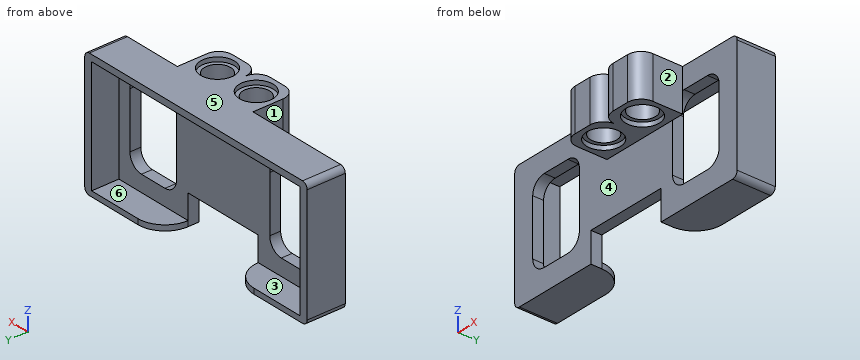
from build123d import *

# Parameters (mm, degrees)
SKETCH1_W           = 48.2
SKETCH1_H           = 23.2
BOSS_EXTRUDE1_DEPTH = 10
SKETCH2_W           = 46.2
SKETCH2_H           = 21.2
CUT_EXTRUDE1_DEPTH  = 8
SKETCH3_W           = 11.2
SKETCH3_H           = 5
CUT_EXTRUDE2_DEPTH  = 10
SKETCH4_W           = 48.2
SKETCH4_H           = 23.2
CUT_EXTRUDE3_DEPTH  = 3
SKETCH5_W           = 8.2
SKETCH5_H           = 7.76
BOSS_EXTRUDE2_DEPTH = 8
SKETCH6_R           = 3.1
CUT_EXTRUDE4_DEPTH  = 0.8
SKETCH7_R           = 2.4
CUT_EXTRUDE5_DEPTH  = 10
SKETCH8_W           = 46.2
SKETCH8_H           = 20.3
CUT_EXTRUDE6_DEPTH  = 5
SKETCH9_W           = 45.4
SKETCH9_H           = 20.3
CUT_EXTRUDE8_DEPTH  = 5
CUT_EXTRUDE9_START  = -0.8
SKETCH10_R          = 3.1
CUT_EXTRUDE9_DEPTH  = 0.8
SKETCH11_W          = 15.2
SKETCH11_H          = 5.5
CUT_EXTRUDE10_DEPTH = 10
CUT_EXTRUDE11_DEPTH = 10
FILLET1_R           = 1
FILLET2_R           = 1
FILLET3_R           = 1
FILLET4_R           = 1
FILLET5_R           = 2.5
FILLET6_R           = 2.5
FILLET7_R           = 5
FILLET8_R           = 5
SKETCH13_W          = 21.2
SKETCH13_H          = 5
BOSS_EXTRUDE3_DEPTH = 0.5
SKETCH14_W          = 21.2
SKETCH14_H          = 5
BOSS_EXTRUDE4_DEPTH = 0.5
SKETCH16_W          = 45.2
SKETCH16_H          = 5
BOSS_EXTRUDE5_DEPTH = 0.2
MIRROR4_START       = 13.310407833
MIRROR4_OUTLINE_R   = 2.4
MIRROR4_DEPTH       = 6.16
MIRROR4_START_2     = 12.510407833
MIRROR4_2_OUTLINE_R = 3.1
MIRROR4_2_DEPTH     = 7.76


# Read off the part's stored shape, not the designer's step: Mirror4
with BuildPart() as part:
    # Sketch1 → Boss-Extrude1 (new body)
    with BuildSketch(Plane(origin=(0, 0, 0), x_dir=(1, 0, 0), z_dir=(0, 1, 0))):
        with Locations((-8.956036835, -8.670407833)):
            Rectangle(SKETCH1_W, SKETCH1_H)
    extrude(amount=BOSS_EXTRUDE1_DEPTH)

    # Sketch2 → Cut-Extrude1 (cut)
    with BuildSketch(Plane(origin=(0, 10, 0), x_dir=(1, 0, 0), z_dir=(0, 1, 0))):
        with Locations((-8.956036835, -8.670407833)):
            Rectangle(SKETCH2_W, SKETCH2_H)
    extrude(amount=-CUT_EXTRUDE1_DEPTH, mode=Mode.SUBTRACT)

    # Sketch3 → Cut-Extrude2 (cut)
    with BuildSketch(Plane(origin=(0, 10, 0), x_dir=(1, 0, 0), z_dir=(0, 1, 0))):
        with Locations((-8.956036835, 0.429592167)):
            Rectangle(SKETCH3_W, SKETCH3_H)
    extrude(amount=-CUT_EXTRUDE2_DEPTH, mode=Mode.SUBTRACT)

    # Sketch4 → Cut-Extrude3 (cut)
    with BuildSketch(Plane(origin=(0, 10, 0), x_dir=(1, 0, 0), z_dir=(0, 1, 0))):
        with Locations((-8.956036835, -8.670407833)):
            Rectangle(SKETCH4_W, SKETCH4_H)
    extrude(amount=-CUT_EXTRUDE3_DEPTH, mode=Mode.SUBTRACT)

    # Sketch5 → Boss-Extrude2 (add)
    with BuildSketch(Plane(origin=(0, 0, 0), x_dir=(-1, 0, 0), z_dir=(0, -1, 0))):
        with Locations((8.956036835, -16.390407833)):
            Rectangle(SKETCH5_W, SKETCH5_H)
    extrude(amount=BOSS_EXTRUDE2_DEPTH)

    # Sketch6 → Cut-Extrude4 (cut)
    with BuildSketch(Plane.XY.offset(20.270407833)):
        with Locations((-9.056036835, -4)):
            Circle(SKETCH6_R)
    extrude(amount=-CUT_EXTRUDE4_DEPTH, mode=Mode.SUBTRACT)

    # Sketch7 → Cut-Extrude5 (cut)
    with BuildSketch(Plane.XY.offset(19.470407833)):
        with Locations((-9.056036835, -4)):
            Circle(SKETCH7_R)
    extrude(amount=-CUT_EXTRUDE5_DEPTH, mode=Mode.SUBTRACT)

    # Sketch8 → Cut-Extrude6 (cut)
    with BuildSketch(Plane(origin=(0, 7, 0), x_dir=(1, 0, 0), z_dir=(0, 1, 0))):
        with Locations((-8.956036835, -8.720407833)):
            Rectangle(SKETCH8_W, SKETCH8_H)
    extrude(amount=-CUT_EXTRUDE6_DEPTH, mode=Mode.SUBTRACT)

    # Sketch9 → Cut-Extrude8 (cut)
    with BuildSketch(Plane(origin=(0, 7, 0), x_dir=(1, 0, 0), z_dir=(0, 1, 0))):
        with Locations((-8.956036835, -8.720407833)):
            Rectangle(SKETCH9_W, SKETCH9_H)
    extrude(amount=-CUT_EXTRUDE8_DEPTH, mode=Mode.SUBTRACT)

    # Sketch10 → Cut-Extrude9 (cut)
    with BuildSketch(Plane(origin=(0, 0, 12.510407833), x_dir=(-1, 0, 0), z_dir=(0, 0, -1)).offset(CUT_EXTRUDE9_START)):
        with Locations(Location((9.056036835, -4, 0), (0, 0, 180))):
            Circle(SKETCH10_R)
    extrude(amount=CUT_EXTRUDE9_DEPTH, mode=Mode.SUBTRACT)

    # Sketch11 → Cut-Extrude10 (cut)
    with BuildSketch(Plane(origin=(0, 7, 0), x_dir=(1, 0, 0), z_dir=(0, 1, 0))):
        with Locations((-8.956036835, 0.179592167)):
            Rectangle(SKETCH11_W, SKETCH11_H)
    extrude(amount=-CUT_EXTRUDE10_DEPTH, mode=Mode.SUBTRACT)

    # Sketch12 → Cut-Extrude11 (cut)
    with BuildSketch(Plane(origin=(0, 2, 0), x_dir=(1, 0, 0), z_dir=(0, 1, 0))):
        with BuildLine():
            Line((8.743963165, -16.370407833), (3.643963165, -16.370407833))
            ThreePointArc((3.643963165, -16.370407833), (1.876196212, -15.638174786), (1.143963165, -13.870407833))
            Line((1.143963165, -13.870407833), (1.143963165, -3.570407833))
            ThreePointArc((1.143963165, -3.570407833), (1.876196212, -1.80264088), (3.643963165, -1.070407833))
            Line((3.643963165, -1.070407833), (8.743963165, -1.070407833))
            ThreePointArc((8.743963165, -1.070407833), (10.511730118, -1.80264088), (11.243963165, -3.570407833))
            Line((11.243963165, -3.570407833), (11.243963165, -13.870407833))
            ThreePointArc((11.243963165, -13.870407833), (10.511730118, -15.638174786), (8.743963165, -16.370407833))
        make_face()
        with BuildLine():
            Line((-21.556036835, -16.370407833), (-26.656036835, -16.370407833))
            ThreePointArc((-26.656036835, -16.370407833), (-28.423803788, -15.638174786), (-29.156036835, -13.870407833))
            Line((-29.156036835, -13.870407833), (-29.156036835, -3.570407833))
            ThreePointArc((-29.156036835, -3.570407833), (-28.423803788, -1.80264088), (-26.656036835, -1.070407833))
            Line((-26.656036835, -1.070407833), (-21.556036835, -1.070407833))
            ThreePointArc((-21.556036835, -1.070407833), (-19.788269882, -1.80264088), (-19.056036835, -3.570407833))
            Line((-19.056036835, -3.570407833), (-19.056036835, -13.870407833))
            ThreePointArc((-19.056036835, -13.870407833), (-19.788269882, -15.638174786), (-21.556036835, -16.370407833))
        make_face()
    extrude(amount=-CUT_EXTRUDE11_DEPTH, mode=Mode.SUBTRACT)

    # Fillet1
    fillet1_edges = [part.edges().sort_by_distance(p)[0] for p in [
        (15.143963165, 3.5, -2.929592167),
    ]]
    fillet(fillet1_edges, radius=FILLET1_R)

    # Fillet2
    fillet2_edges = [part.edges().sort_by_distance(p)[0] for p in [
        (15.143963165, 3.5, 20.270407833),
    ]]
    fillet(fillet2_edges, radius=FILLET2_R)

    # Fillet3
    fillet3_edges = [part.edges().sort_by_distance(p)[0] for p in [
        (-33.056036835, 3.5, 20.270407833),
    ]]
    fillet(fillet3_edges, radius=FILLET3_R)

    # Fillet4
    fillet4_edges = [part.edges().sort_by_distance(p)[0] for p in [
        (-33.056036835, 3.5, -2.929592167),
    ]]
    fillet(fillet4_edges, radius=FILLET4_R)

    # Fillet5
    fillet5_edges = [part.edges().sort_by_distance(p)[0] for p in [
        (-13.056036835, -8, 16.390407833),
    ]]
    fillet(fillet5_edges, radius=FILLET5_R)

    # Fillet6
    fillet6_edges = [part.edges().sort_by_distance(p)[0] for p in [
        (-4.856036835, -8, 16.390407833),
    ]]
    fillet(fillet6_edges, radius=FILLET6_R)

    # Fillet7
    fillet7_edges = [part.edges().sort_by_distance(p)[0] for p in [
        (-1.356036835, 7, -2.429592167),
    ]]
    fillet(fillet7_edges, radius=FILLET7_R)

    # Fillet8
    fillet8_edges = [part.edges().sort_by_distance(p)[0] for p in [
        (-16.556036835, 7, -2.429592167),
    ]]
    fillet(fillet8_edges, radius=FILLET8_R)

    # Sketch13 → Boss-Extrude3 (add)
    with BuildSketch(Plane.ZY.offset(-14.143963165)):
        with Locations((8.670407833, 4.5)):
            Rectangle(SKETCH13_W, SKETCH13_H)
    extrude(amount=BOSS_EXTRUDE3_DEPTH)

    # Sketch14 → Boss-Extrude4 (add)
    with BuildSketch(Plane(origin=(-32.056036835, 0, 0), x_dir=(0, 0, -1), z_dir=(1, 0, 0))):
        with Locations((-8.670407833, 4.5)):
            Rectangle(SKETCH14_W, SKETCH14_H)
    extrude(amount=BOSS_EXTRUDE4_DEPTH)

    # Sketch16 → Boss-Extrude5 (add)
    with BuildSketch(Plane(origin=(0, 0, 19.270407833), x_dir=(-1, 0, 0), z_dir=(0, 0, -1))):
        with Locations((8.956036835, 4.5)):
            Rectangle(SKETCH16_W, SKETCH16_H)
    extrude(amount=BOSS_EXTRUDE5_DEPTH)

    # Mirror4 outline → Mirror4 (add)
    with BuildSketch(Plane.XY.offset(MIRROR4_START)):
        with BuildLine():
            ThreePointArc((-4.856036835, -5.5), (-4.123803788, -7.267766953), (-2.356036835, -8))
            Line((-2.356036835, -8), (0.843963165, -8))
            ThreePointArc((0.843963165, -8), (2.611730118, -7.267766953), (3.343963165, -5.5))
            Line((3.343963165, -5.5), (3.343963165, 0))
            Line((3.343963165, 0), (-4.856036835, 0))
            Line((-4.856036835, 0), (-4.856036835, -5.5))
        make_face()
        with Locations((-0.656036835, -4)):
            Circle(MIRROR4_OUTLINE_R, mode=Mode.SUBTRACT)
    extrude(amount=MIRROR4_DEPTH)

    # Mirror4 2 outline → Mirror4 2 (add)
    with BuildSketch(Plane.XY.offset(MIRROR4_START_2)):
        with BuildLine():
            ThreePointArc((-4.856036835, -5.5), (-4.123803788, -7.267766953), (-2.356036835, -8))
            Line((-2.356036835, -8), (0.843963165, -8))
            ThreePointArc((0.843963165, -8), (2.611730118, -7.267766953), (3.343963165, -5.5))
            Line((3.343963165, -5.5), (3.343963165, 0))
            Line((3.343963165, 0), (-4.856036835, 0))
            Line((-4.856036835, 0), (-4.856036835, -5.5))
        make_face()
        with Locations((-0.656036835, -4)):
            Circle(MIRROR4_2_OUTLINE_R, mode=Mode.SUBTRACT)
    extrude(amount=MIRROR4_2_DEPTH)


solid = part.part
Design review of the part built by this model. Coordinates are the model's own, in mm. Face numbers are marked on the shaded views. A direction names the side the tool comes from. Round coordinates to 2 decimals unless told otherwise and drop trailing zeros. Write each loop counter-clockwise with the first axis right and the second up, starting at its lowest first coordinate (ties: lowest second). Pieces come first, ordered by that corner, then holes. Notation, with made-up numbers: (65, 78) -> (80, 78) arc R36 cw to (80, 114) -> close; hole circle Ø1 at (74, 18.5). An arc over 180 degrees is marked (long way). One line per item, written item: value. Start each with the question number.
Q1. Add section B-B (z = 11). Give the boundary of the cut face in (x, y), then the cut area to 3 significant figures.
Q2. Insertion check: P1, Ø5.5, axis at x = -9.06, y = -4, coming from the -Z side; P2, Ø4, axis at x = -2.5, y = -5.5, coming from the -Z side; P3, Ø5, axis at x = -9.06, y = -4, coming from the +Z side. Each pin has a flat end and moves straight along its axis. Give the tip position at first contact, or say it passes through.
Q3. The part is to be moulded in two halves that separate along Z. For the marked faces 4, 5 and 6, say which applies: pulls with the +Z half, pulls with the -Z half, needs draft (parallel to the pull), parting line crosses it, or undercut.
Q4. To check wall thickness, follow probe 1 along X at (y, z) = (3, 17); probe 2 along Y at (x, z) = (-12, 5.5); probe 3 along X at (y, z) = (1, 1). State the ranges of each line that lie inside material, in increasing order.
Q5. Add section A-A (x = -25). Give the boundary of the cut face in (y, z).
Q6. Add section C-C (y = -4). Give the boundary of the cut face in (x, z).
Q7. Add section D-D (z = -1). Give the boundary of the cut face in (x, y), then the cut area to 3 significant figures.
Q8. Tool access review of the marked faces 1, 2 and 3: name each direction out of +Z, -Z, +X, -X, +Y, -Y from which nothing blocks a thin tool from reaching the whole face with its end or side.
Response:
1. outline: (-33.06, 0) -> (-29.16, 0) -> (-29.16, 2) -> (-31.56, 2) -> (-31.56, 7) -> (-33.06, 7) -> close; (-19.06, 0) -> (1.14, 0) -> (1.14, 2) -> (-19.06, 2) -> close; (11.24, 0) -> (15.14, 0) -> (15.14, 7) -> (13.64, 7) -> (13.64, 2) -> (11.24, 2) -> close
1. area: 71.0 mm^2
2. P1: stops at z = 13.31
2. P2: stops at z = 12.51
2. P3: stops at z = 19.47
3. face 4: needs draft
3. face 5: pulls with the +Z half
3. face 6: undercut
4. probe 1: x = -33.06 to -31.56, 13.64 to 15.14
4. probe 2: y = 0 to 2
4. probe 3: x = -33.06 to -16.56, -1.36 to 15.14
5. outline: (0, -2.93) -> (7, -2.93) -> (7, -1.93) -> (2, -1.93) -> (2, 1.07) -> (0, 1.07) -> close; (0, 16.37) -> (2, 16.37) -> (2, 19.07) -> (7, 19.07) -> (7, 20.27) -> (0, 20.27) -> close
6. outline: (-13.06, 12.51) -> (-12.16, 12.51) -> (-12.16, 13.31) -> (-11.46, 13.31) -> (-11.46, 19.47) -> (-12.16, 19.47) -> (-12.16, 20.27) -> (-13.06, 20.27) -> close; (-6.66, 13.31) -> (-5.96, 13.31) -> (-5.96, 12.51) -> (-3.76, 12.51) -> (-3.76, 13.31) -> (-3.06, 13.31) -> (-3.06, 19.47) -> (-3.76, 19.47) -> (-3.76, 20.27) -> (-5.96, 20.27) -> (-5.96, 19.47) -> (-6.66, 19.47) -> close; (1.74, 13.31) -> (2.44, 13.31) -> (2.44, 12.51) -> (3.34, 12.51) -> (3.34, 20.27) -> (2.44, 20.27) -> (2.44, 19.47) -> (1.74, 19.47) -> close
7. outline: (-33.06, 0) -> (-16.56, 0) -> (-16.56, 2) -> (-31.56, 2) -> (-31.56, 7) -> (-33.06, 7) -> close; (-1.36, 0) -> (15.14, 0) -> (15.14, 7) -> (13.64, 7) -> (13.64, 2) -> (-1.36, 2) -> close
7. area: 81.0 mm^2
8. face 1: +Z, -Z, -X, -Y
8. face 2: +Z, -Z, +X, -Y
8. face 3: +Y
